Can you work these out from the model? Positions are in its coordinate system, mm. Give positions to 0.01 mm unless a question says otherwise; leave off trailing zeros. Order: outer loops, then holes, each group sorted by start corner. A loop starts at its lowest first (then second) coordinate and runs counter-clockwise, first axis right, second up. Notation, with made-up numbers: (-23, 71.25) - (-3, 71.25) arc R32 cw to (-3, 101.25) - close; hole circle Ø5 at (41.5, -17). An arc over 180 degrees is marked (long way). Use one line per item in the form item = value. Start each with the question number.
1) For pin 1 (1.5 mm diameter, centred on y = 1.5, z = -19.5, fed in from +X); pin 2 (0.9 mm diameter, centred on x = -20, y = 2, fed in from -Z); pin 3 (0.9 mm diameter, centred on x = -17.5, y = 1, fed in from +Z); pin 4 (1.2 mm diameter, centred on x = 0, z = 10.7, fed in from -Y), each with a flat end and sliding along its axis, tell me the tip position at first contact or that it passes through.
2) Suppose I cut it at C-C, the plane y = 2.5. State how many separate pieces and enclosed holes the cut face has, and give its area (3 significant figures).
3) Suppose I cut it at B-B, the plane x = -34. Write out the boundary of the cut face in (y, z), and give its area (3 significant figures).
4) Suppose I cut it at A-A, the plane z = 27. Write out the boundary of the cut face in (x, y), and give its area (3 significant figures).
5) Please list where these lines run through material, in increasing order: probe 1 along Z at (x, y) = (18, 0.2); probe 2 along X at (y, z) = (2.2, 15.5); probe 3 along X at (y, z) = (1.2, 27.5).
6) Suppose I cut it at D-D, the plane x = 8. Write out the boundary of the cut face in (y, z), and give its area (3 significant figures).
```python
from build123d import *

# Parameters (mm, degrees)
SKETCH1_R           = 1.65
SKETCH1_R_2         = 1
SKETCH1_R_3         = 0.75
BOSS_EXTRUDE1_DEPTH = 3
SKETCH2_W           = 4
SKETCH2_H           = 7.5
SKETCH2_W_2         = 7.5
SKETCH2_H_2         = 4
SKETCH2_H_3         = 7.405429953
CUT_EXTRUDE1_DEPTH  = 4


with BuildPart() as part:
    # Sketch1 → Boss-Extrude1 (new body)
    with BuildSketch(Plane(origin=(0, 0, 0), x_dir=(1, 0, 0), z_dir=(0, 1, 0))):
        with BuildLine():
            Line((-26.64113361, 37.5), (-23, 37.5))
            Line((-23, 37.5), (-23, 32.5))
            Line((-23, 32.5), (23, 32.5))
            Line((23, 32.5), (23, 37.5))
            Line((23, 37.5), (26.64113361, 37.5))
            ThreePointArc((26.64113361, 37.5), (46, 0), (26.64113361, -37.5))
            Line((26.64113361, -37.5), (23, -37.5))
            Line((23, -37.5), (23, -32.405429953))
            Line((23, -32.405429953), (-23.13261865, -32.405429953))
            Line((-23.13261865, -32.405429953), (-23.13261865, -37.405429953))
            Line((-23.13261865, -37.405429953), (-26.77375226, -37.405429953))
            ThreePointArc((-26.77375226, -37.405429953), (-45.999927904, 0.081442004), (-26.64113361, 37.5))
        make_face()
        with Locations((34, -15)):
            Circle(SKETCH1_R, mode=Mode.SUBTRACT)
        with Locations((34, 15)):
            Circle(SKETCH1_R, mode=Mode.SUBTRACT)
        with Locations((-34, 15)):
            Circle(SKETCH1_R, mode=Mode.SUBTRACT)
        with Locations((-34, -15)):
            Circle(SKETCH1_R, mode=Mode.SUBTRACT)
        Circle(SKETCH1_R_2, mode=Mode.SUBTRACT)
        with Locations((0, 8.7)):
            Circle(SKETCH1_R_3, mode=Mode.SUBTRACT)
        with Locations((0, 10.7)):
            Circle(SKETCH1_R_3, mode=Mode.SUBTRACT)
        with Locations((0, 12.7)):
            Circle(SKETCH1_R_3, mode=Mode.SUBTRACT)
        with Locations((0, 6.7)):
            Circle(SKETCH1_R_3, mode=Mode.SUBTRACT)
        with Locations((0, 4.7)):
            Circle(SKETCH1_R_3, mode=Mode.SUBTRACT)
        with Locations((0, -12.7)):
            Circle(SKETCH1_R_3, mode=Mode.SUBTRACT)
        with Locations((0, -10.7)):
            Circle(SKETCH1_R_3, mode=Mode.SUBTRACT)
        with Locations((0, -8.7)):
            Circle(SKETCH1_R_3, mode=Mode.SUBTRACT)
        with Locations((0, -6.7)):
            Circle(SKETCH1_R_3, mode=Mode.SUBTRACT)
        with Locations((0, -4.7)):
            Circle(SKETCH1_R_3, mode=Mode.SUBTRACT)
    extrude(amount=BOSS_EXTRUDE1_DEPTH)

    # Sketch2 → Cut-Extrude1 (cut, through all)
    with BuildSketch(Plane(origin=(0, 3, 0), x_dir=(1, 0, 0), z_dir=(0, 1, 0))):
        with Locations((-14.6, 28.75)):
            Rectangle(SKETCH2_W, SKETCH2_H)
        Polygon((-12.6, 25), (-16.6, 25), (-18.35, 25), (-18.35, 21), (-10.85, 21), (-10.85, 25), align=None)
        with Locations((14.6, 28.75)):
            Rectangle(SKETCH2_W, SKETCH2_H)
        with Locations((14.6, 23)):
            Rectangle(SKETCH2_W_2, SKETCH2_H_2)
        with Locations((-14.6, -23)):
            Rectangle(SKETCH2_W_2, SKETCH2_H_2)
        with Locations((-14.6, -28.702714977)):
            Rectangle(SKETCH2_W, SKETCH2_H_3)
        Polygon((12.6, -25), (16.6, -25), (18.35, -25), (18.35, -21), (10.85, -21), (10.85, -25), align=None)
        with Locations((14.6, -28.702714977)):
            Rectangle(SKETCH2_W, SKETCH2_H_3)
    extrude(amount=-CUT_EXTRUDE1_DEPTH, mode=Mode.SUBTRACT)


solid = part.part
```
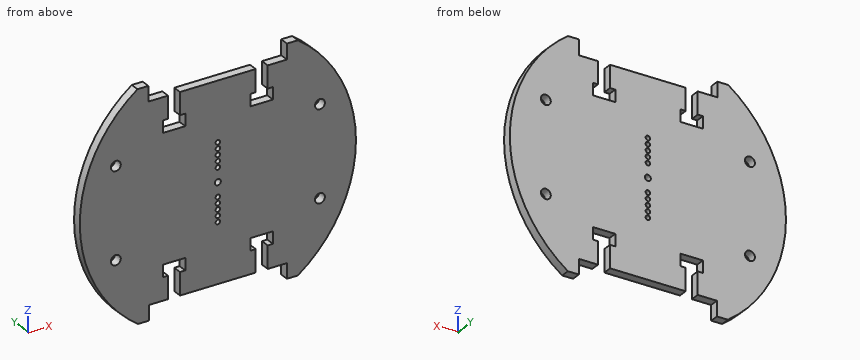
Result sheet:
q1.pin_1 = 42.01
q1.pin_2 = -32.5
q1.pin_3 = 32.41
q1.pin_4 = through
q2.separate_pieces = 1
q2.enclosed_holes = 15
q2.area = 5,270 mm²
q3.outline = (0, -30.98) - (3, -30.98) - (3, -16.65) - (0, -16.65) - close; (0, -13.35) - (3, -13.35) - (3, 13.35) - (0, 13.35) - close; (0, 16.65) - (3, 16.65) - (3, 30.98) - (0, 30.98) - close
q3.area = 166 mm²
q4.outline = (-37.24, 0) - (-16.6, 0) - (-16.6, 3) - (-37.24, 3) - close; (-12.6, 0) - (12.6, 0) - (12.6, 3) - (-12.6, 3) - close; (16.6, 0) - (37.24, 0) - (37.24, 3) - (16.6, 3) - close
q4.area = 199 mm²
q5.probe_1 = -32.5 to -25, -21 to 21, 25 to 32.41
q5.probe_2 = -43.31 to -35.57, -32.43 to 32.43, 35.57 to 43.31
q5.probe_3 = -36.87 to -16.6, -12.6 to 12.6, 16.6 to 36.87
q6.outline = (0, -32.5) - (3, -32.5) - (3, 32.41) - (0, 32.41) - close
q6.area = 195 mm²
